```python
from build123d import *

# Parameters (mm, degrees)
F1_DEPTH = 0.6
F2_SIZE  = 5


with BuildPart() as f1:
    # F0 (on Top) → F1 (new body)
    with BuildSketch(Plane.XY):
        Polygon((-48, 14), (-48, 0), (-48, -14), (-33, -14), (-33, -39), (-53, -39), (-53, -54), (-18, -54), (-18, -23), (0, -23), (18, -23), (18, -54), (53, -54), (53, -39), (33, -39), (33, -14), (48, -14), (48, 0), (48, 14), (33, 14), (33, 39), (53, 39), (53, 54), (18, 54), (18, 23), (-18, 23), (-18, 54), (-53, 54), (-53, 39), (-33, 39), (-33, 14), align=None)
    extrude(amount=F1_DEPTH)

    # F2
    f2_edges = [f1.edges().sort_by_distance(p)[0] for p in [
        (-48, 14, 0.3),
        (-48, -14, 0.3),
        (48, 14, 0.3),
        (48, -14, 0.3),
    ]]
    chamfer(f2_edges, length=F2_SIZE)


solid = f1.part
```
Verification items for the finished model (mm, model axes). A direction names the side the tool comes from. Give positions to 0.01 mm unless a question says otherwise; leave off trailing zeros. Order: outer loops, then holes, each group sorted by start corner. A loop starts at its lowest first (then second) coordinate and runs counter-clockwise, first axis right, second up. Notation, with made-up numbers: (-29.5, 35) - (-4.5, 35) arc R15 cw to (-4.5, 57) - close; hole circle Ø4 at (77.25, 8). An arc over 180 degrees is marked (long way). Answer as CSV lines item,"result". Start each with the question number.
Item 1: Access from +Z, -Z, +X, -X, +Y, -Y to the whole of each face (thin tool, end or side, straight path). Record for faces 1 (the face through (-1, 1, 0)), 2 (the face through (-45.5, -11.5, 0.3)), 3 (the face through (45.5, 11.5, 0.3)).
Item 2: Section check A-A, the plane y = -32.5. Record the boundary of the cut face in (x, z).
Item 3: Material ranges on L1, parallel to Y at x = 40.5, z = 0.5; L2, parallel to X at y = -44, z = 0.15; L3, parallel to Y at x = -46.5, z = 0.2, recorded low to high.
Item 4: Section check B-B, the plane x = 39. Record the boundary of the cut face in (y, z).
Item 5: Section check D-D, the plane x = -45. Record the boundary of the cut face in (y, z), plus the area to 3 significant figures.
Filled in:
1,face 1,"-Z, +X, -X, +Y, -Y"
1,face 2,"+Z, -Z, -X"
1,face 3,"+Z, -Z, +X"
2,outline,"(-33, 0) - (-18, 0) - (-18, 0.6) - (-33, 0.6) - close; (18, 0) - (33, 0) - (33, 0.6) - (18, 0.6) - close"
3,L1,"-54 to -39, -14 to 14, 39 to 54"
3,L2,"-53 to -18, 18 to 53"
3,L3,"-54 to -39, -10.5 to 10.5, 39 to 54"
4,outline,"(-54, 0) - (-39, 0) - (-39, 0.6) - (-54, 0.6) - close; (-14, 0) - (14, 0) - (14, 0.6) - (-14, 0.6) - close; (39, 0) - (54, 0) - (54, 0.6) - (39, 0.6) - close"
5,outline,"(-54, 0) - (-39, 0) - (-39, 0.6) - (-54, 0.6) - close; (-12, 0) - (12, 0) - (12, 0.6) - (-12, 0.6) - close; (39, 0) - (54, 0) - (54, 0.6) - (39, 0.6) - close"
5,area,"32.4 mm^2"
